Input: part model. Units: mm. Frame: model coordinates. Face numbers are marked on the shaded views. A direction names the side the tool comes from. Give positions to 0.01 mm unless a question says otherwise; leave off trailing zeros. Order: outer loops, then holes, each group sorted by start corner. A loop starts at its lowest first (then second) coordinate and runs counter-clockwise, first axis right, second up. Notation, with made-up numbers: (61, -15.75) - (74, -15.75) arc R32 ccw to (74, 18.25) - close; hole circle Ø3 at (-37.5, -30). An arc over 180 degrees is marked (long way). Use a Markdown table: item, result.
from build123d import *

# Parameters (mm, degrees)
F0_W      = 65.7
F0_H      = 65.7
F1_DEPTH  = 3.175
F2_W      = 65.7
F2_H      = 99
F2_W_2    = 53
F2_H_2    = 86.3
F3_DEPTH  = 65.7
F4_DEPTH  = 6.35
F5_R      = 3.429
F6_DEPTH  = 65.701
F7_R      = 5.08
F8_W      = 53
F8_H      = 6
F9_DEPTH  = 5
F10_R     = 1.5875
F10_R_2   = 1.55
F11_DEPTH = 10


# Not quite as in the source:
# - a length typed as a fraction of an inch, garbled in the dataset ("3 / 203.2 mm" for 3/8 in), is restored


with BuildPart() as f1:
    # F0 (on Top) → F1 (new body)
    with BuildSketch(Plane.XY):
        Rectangle(F0_W, F0_H)
        Polygon((26.5, 26.5), (26.5, -26.5), (-26.5, -26.5), (-26.5, -24.0082931455), (-26.5, 26.5), align=None, mode=Mode.SUBTRACT)
    extrude(amount=F1_DEPTH)

    # F2 (on face) → F3 (join)
    with BuildSketch(Plane.XZ.offset(32.85)):
        with Locations((0, -49.5)):
            Rectangle(F2_W, F2_H)
        with Locations((0, -49.5)):
            Rectangle(F2_W_2, F2_H_2, mode=Mode.SUBTRACT)
    extrude(amount=-F3_DEPTH)

    # F4 (cut): faces of the model
    f4_faces = [f1.faces().sort_by_distance(p)[0] for p in [
        (0, 0, 0),
        (0, 0, 0),
    ]]
    extrude(f4_faces, amount=-F4_DEPTH, mode=Mode.SUBTRACT)

    # F5 (on face) → F6 (cut, through all)
    with BuildSketch(Plane(origin=(-32.85, 0, 0), x_dir=(0, -1, 0), z_dir=(-1, 0, 0))):
        with Locations((0, -56.35)):
            Circle(F5_R)
        with Locations((0, -6.35)):
            Circle(F5_R)
        with BuildLine():
            ThreePointArc((22.85, -15.325), (21.8248737342, -12.8501262658), (19.35, -11.825))
            Line((19.35, -11.825), (13.35, -11.825))
            ThreePointArc((13.35, -11.825), (10.8751262658, -12.8501262658), (9.85, -15.325))
            Line((9.85, -15.325), (9.85, -80.325))
            ThreePointArc((9.85, -80.325), (10.8751262658, -82.7998737342), (13.35, -83.825))
            Line((13.35, -83.825), (19.35, -83.825))
            ThreePointArc((19.35, -83.825), (21.8248737342, -82.7998737342), (22.85, -80.325))
            Line((22.85, -80.325), (22.85, -15.325))
        make_face()
        with BuildLine():
            ThreePointArc((-8.86, -15.325), (-9.8851262658, -12.8501262658), (-12.36, -11.825))
            Line((-12.36, -11.825), (-19.36, -11.825))
            ThreePointArc((-19.36, -11.825), (-21.8348737342, -12.8501262658), (-22.86, -15.325))
            Line((-22.86, -15.325), (-22.86, -80.325))
            ThreePointArc((-22.86, -80.325), (-21.8348737342, -82.7998737342), (-19.36, -83.825))
            Line((-19.36, -83.825), (-12.36, -83.825))
            ThreePointArc((-12.36, -83.825), (-9.8851262658, -82.7998737342), (-8.86, -80.325))
            Line((-8.86, -80.325), (-8.86, -15.325))
        make_face()
    extrude(amount=-F6_DEPTH, mode=Mode.SUBTRACT)

    # F7
    f7_edges = [f1.edges().sort_by_distance(p)[0] for p in [
        (0, -32.85, 3.175),
        (32.85, 0, 3.175),
        (0, 32.85, 3.175),
        (-32.85, 0, 3.175),
        (32.85, 32.85, -47.9125),
        (32.85, -32.85, -47.9125),
        (-32.85, -32.85, -47.9125),
        (-32.85, 32.85, -47.9125),
        (0, 32.85, -99),
        (-32.85, 0, -99),
        (32.85, 0, -99),
        (0, -32.85, -99),
    ]]
    fillet(f7_edges, radius=F7_R)

    # F8 (on face) → F9 (join)
    with BuildSketch(Plane.XZ.offset(32.85)):
        with Locations((0, -37.15)):
            Rectangle(F8_W, F8_H)
    extrude(amount=-F9_DEPTH)

    # F10 (on face) → F11 (cut)
    with BuildSketch(Plane(origin=(0, 0, -99), x_dir=(1, 0, 0), z_dir=(0, 0, -1))):
        with Locations((0, 20.3174948692)):
            Circle(F10_R)
        with Locations((-14.0181705356, 1.279)):
            Circle(F10_R_2)
        with Locations((14.0181705356, 1.279)):
            Circle(F10_R_2)
        with Locations((-14.0181705356, 6.279)):
            Circle(F10_R_2)
        with Locations((-14.0181705356, -3.721)):
            Circle(F10_R_2)
        with Locations((14.0181705356, 6.279)):
            Circle(F10_R_2)
        with Locations((14.0181705356, -3.721)):
            Circle(F10_R_2)
        with Locations((0, -22.6024445146)):
            Circle(F10_R)
    extrude(amount=-F11_DEPTH, mode=Mode.SUBTRACT)


solid = f1.part
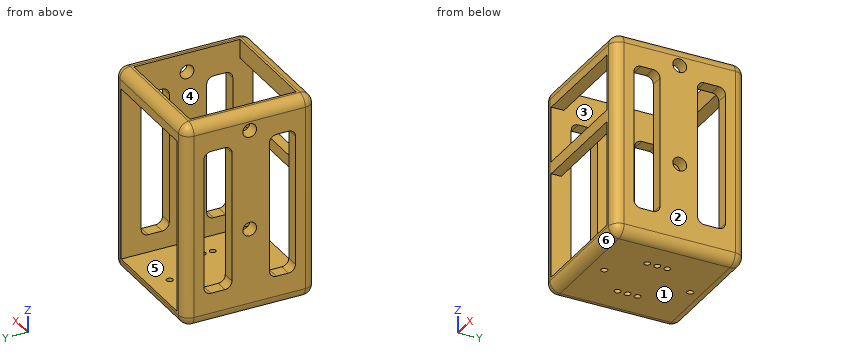
1. Section query C-C (y = -24.5). Return loops of the section in (x, z) (3 decimals).
Response:
| item | result |
|---|---|
| outline | (-32.85, -93.92) arc R5.08 ccw to (-27.77, -99) - (27.77, -99) arc R5.08 ccw to (32.85, -93.92) - (32.85, -1.905) arc R5.08 ccw to (27.77, 3.175) - (26.5, 3.175) - (26.5, -92.65) - (-26.5, -92.65) - (-26.5, 3.175) - (-27.77, 3.175) arc R5.08 ccw to (-32.85, -1.905) - close |
2. Material intervals for line 1 along Z through (x, y) = (-27, 0) (3 decimals); line 2 along X through (y, z) = (26, -39.5), sorted ascending.
Response:
| item | result |
|---|---|
| line 1 | z = -99 to -59.779, -52.921 to -9.779, -2.921 to 3.175 |
| line 2 | x = -32.85 to -26.5, 26.5 to 32.85 |
3. Mould query, pull axis X, two halves, no side actions, for the marked faces 1, 2 and 3. Classes: pulls with the +X half, pulls with the -X half, needs draft (parallel to the pull), parting line crosses it, or undercut.
Response:
| item | result |
|---|---|
| face 1 | needs draft |
| face 2 | pulls with the +X half |
| face 3 | undercut |
4. Section query B-B (z = -62). Return loops of the section in (x, y).
Response:
| item | result |
|---|---|
| outline | (-32.85, -27.77) arc R5.08 ccw to (-27.77, -32.85) - (-26.5, -32.85) - (-26.5, -22.85) - (-32.85, -22.85) - close; (-32.85, -9.85) - (-26.5, -9.85) - (-26.5, 8.86) - (-32.85, 8.86) - close; (-32.85, 22.86) - (-26.5, 22.86) - (-26.5, 32.85) - (-27.77, 32.85) arc R5.08 ccw to (-32.85, 27.77) - close; (26.5, -32.85) - (27.77, -32.85) arc R5.08 ccw to (32.85, -27.77) - (32.85, -22.85) - (26.5, -22.85) - close; (26.5, -9.85) - (32.85, -9.85) - (32.85, 8.86) - (26.5, 8.86) - close; (26.5, 22.86) - (32.85, 22.86) - (32.85, 27.77) arc R5.08 ccw to (27.77, 32.85) - (26.5, 32.85) - close |
5. Set-up query: the marked faces 4, 5 and 6. Return all of +Z, -Z, +X, -X, +Y, -Y with unobstructed straight access to the full face (end or side cutting, diameter ignored); none if empty.
Response:
| item | result |
|---|---|
| face 4 | none |
| face 5 | +Y, -Y |
| face 6 | -Z, +X, -X, -Y |
6. Section query A-A (x = 7.5). Return loops of the section in (y, z) (3 decimals).
Response:
| item | result |
|---|---|
| outline | (-32.85, -93.92) arc R5.08 ccw to (-27.77, -99) - (27.77, -99) arc R5.08 ccw to (32.85, -93.92) - (32.85, -92.65) - (-32.85, -92.65) - close; (-32.85, -40.15) - (-27.85, -40.15) - (-27.85, -34.15) - (-32.85, -34.15) - close; (-32.85, -6.35) - (-26.5, -6.35) - (-26.5, 3.175) - (-27.77, 3.175) arc R5.08 ccw to (-32.85, -1.905) - close; (26.5, -6.35) - (32.85, -6.35) - (32.85, -1.905) arc R5.08 ccw to (27.77, 3.175) - (26.5, 3.175) - close |
7. Section query D-D (x = 0). Return loops of the section in (y, z) (3 decimals).
Response:
| item | result |
|---|---|
| outline | (-32.85, -93.92) arc R5.08 ccw to (-27.77, -99) - (-21.905, -99) - (-21.905, -92.65) - (-32.85, -92.65) - close; (-32.85, -40.15) - (-27.85, -40.15) - (-27.85, -34.15) - (-32.85, -34.15) - close; (-32.85, -6.35) - (-26.5, -6.35) - (-26.5, 3.175) - (-27.77, 3.175) arc R5.08 ccw to (-32.85, -1.905) - close; (-18.73, -99) - (21.015, -99) - (21.015, -92.65) - (-18.73, -92.65) - close; (24.19, -99) - (27.77, -99) arc R5.08 ccw to (32.85, -93.92) - (32.85, -92.65) - (24.19, -92.65) - close; (26.5, -6.35) - (32.85, -6.35) - (32.85, -1.905) arc R5.08 ccw to (27.77, 3.175) - (26.5, 3.175) - close |
8. Pin query (flat end, axial travel): pin 1 (3 mm diameter, centred on x = -6, z = -0.5, fed in from +Y); pin 2 (8 mm diameter, centred on x = -0.5, y = 15.5, fed in from +Z); pin 3 (4 mm diameter, centred on y = 0, z = -6.35, fed in from -X); pin 4 (1.9 mm diameter, centred on x = 8, y = 29.5, fed in from -Z). Return the tip coordinate at first contact, or that it passes through.
Response:
| item | result |
|---|---|
| pin 1 | stops at y = 32.85 |
| pin 2 | stops at z = -92.65 |
| pin 3 | passes through |
| pin 4 | stops at z = -98.94 |
